Source: three-view drawing plus pictorial views. Frame: mm from the lowest corner of the part. A direction names the side the tool comes from. Round coordinates to 2 decimals unless told otherwise and drop trailing zeros. Write each loop counter-clockwise with the first axis right and the second up, starting at its lowest first coordinate (ties: lowest second). Pieces come first, ordered by that corner, then holes. Notation, with made-up numbers: (79, -38.5) -> (113, -38.5) arc R7 ccw to (113, -26.5) -> close; hole circle Ø4 at (-21.5, -38.5). An arc over 180 degrees is marked (long way). Put each result on its own line as item: value.
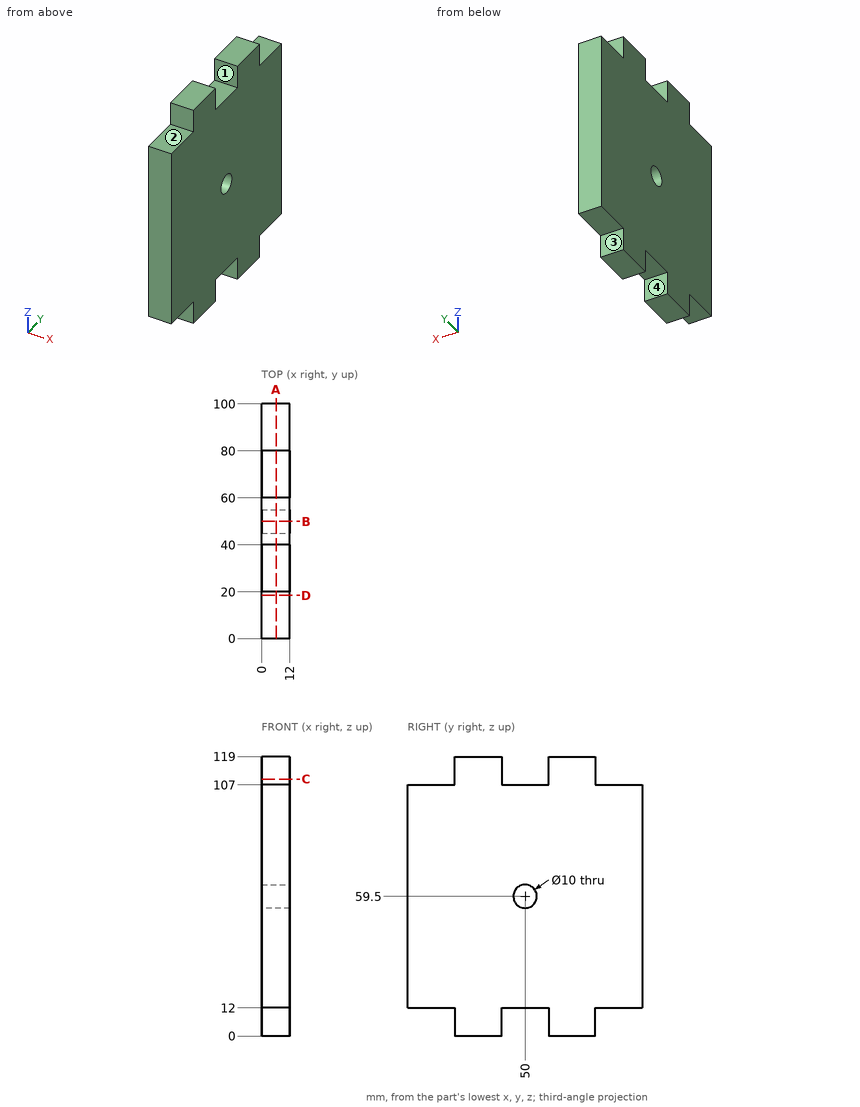
Q1. Pin query (flat end, axial travel): pin 1 (6 mm diameter, centred on x = 3, z = 115, fed in from +Y); pin 2 (6 mm diameter, centred on x = 5, y = 11.5, fed in from +Z); pin 3 (3.5 mm diameter, centred on x = 4, y = 47.5, fed in from -Z). Return the tip coordinate at first contact, or that it passes through.
Ans:
pin 1: stops at y = 80
pin 2: stops at z = 107
pin 3: stops at z = 12
Q2. Material intervals for line 1 (Y direction, x = 4, z = 60); line 2 (Y direction, x = 7.5, z = 10); line 3 (Z direction, x = 6.25, y = 81), sorted ascending. Write a range as [from, to].
Ans:
line 1: y = [0, 45.03], [54.97, 100]
line 2: y = [20, 40], [60, 80]
line 3: z = [12, 107]
Q3. Cut plane C-C on z = 109.5. Output: boundary loops of the cut face in (x, y).
Ans:
outline: (0, 20) -> (12, 20) -> (12, 40) -> (0, 40) -> close; (0, 60) -> (12, 60) -> (12, 80) -> (0, 80) -> close
Q4. Cut plane D-D on y = 18.5. Output: boundary loops of the cut face in (x, z).
Ans:
outline: (0, 12) -> (12, 12) -> (12, 107) -> (0, 107) -> close
Q5. Cut plane B-B on y = 50. Output: boundary loops of the cut face in (x, z).
Ans:
outline: (0, 12) -> (12, 12) -> (12, 54.5) -> (0, 54.5) -> close; (0, 64.5) -> (12, 64.5) -> (12, 107) -> (0, 107) -> close
Q6. Reachability of the marked faces 1, 2, 3 and 4 from +Z, -Z, +X, -X, +Y, -Y: full face, straight path, thin tool, end or side. Return the list, or none.
Ans:
face 1: +Z, +X, -X
face 2: +Z, +X, -X, -Y
face 3: -Z, +X, -X, +Y
face 4: -Z, +X, -X
Q7. Cut plane A-A on x = 6.25. Output: boundary loops of the cut face in (y, z).
Ans:
outline: (0, 12) -> (20, 12) -> (20, 0) -> (40, 0) -> (40, 12) -> (60, 12) -> (60, 0) -> (80, 0) -> (80, 12) -> (100, 12) -> (100, 107) -> (80, 107) -> (80, 119) -> (60, 119) -> (60, 107) -> (40, 107) -> (40, 119) -> (20, 119) -> (20, 107) -> (0, 107) -> close; hole circle Ø10 at (50, 59.5)
